The listing builds one solid part. Answer for the finished solid, in the listing's coordinates (mm). Coordinates: 2 decimals unless noted, no trailing zeros. Write each loop counter-clockwise with the first axis right and the second up, starting at its lowest first coordinate (ties: lowest second). Pieces come first, ordered by that corner, then holes.
Autodesk Inventor part; units mm, degrees
ref_plane "YZ Plane" through (0, 0, 0) normal (1, 0, 0) x (0, 1, 0)
ref_plane "XZ Plane" through (0, 0, 0) normal (0, 1, 0) x (-1, 0, 0)
ref_plane "XY Plane" through (0, 0, 0) normal (0, 0, 1) x (1, 0, 0)
sketch "Sketch1" plane through (0, 0, 0) normal (0, 0, 1) x (1, 0, 0)
  circle A0 centre (0, 0) radius 14.5
  dimension "d6" = 29
extrude "Extrusion3" add sketch "Sketch1" along normal blind 300
sketch "Sketch3" plane through (0, 0, 0) normal (1, 0, 0) x (0, 1, 0)
  line L0 (-7, 295.5461) -> (7, 295.5461)
  line L1 (7, 295.5461) -> (7, 320)
  line L2 (7, 320) -> (-7, 320)
  line L3 (-7, 320) -> (-7, 295.5461)
  line L4 (0, 384) -> (0, -64)
  line L5 (14.5, 300) -> (-14.5, 300)
  point P0 (0, 0)
  point P1 (7, 300)
  point P2 (-7, 300)
  dimension "d9" = 7
  dimension "d10" = 7
  dimension "d11" = 20
extrude "Extrusion4" add sketch "Sketch3" along normal mid plane 10 contours L3 L2 L4 L5 | L4 L2 L1 L5
fillet "Fillet1" radius 2 2 edges at (0, -7, 300) (0, 7, 300)
fillet "Fillet2" radius 5 2 edges at (0, -7, 320) (0, 7, 320)
sketch "Sketch4" plane through (5, 0, 0) normal (1, 0, 0) x (0, 0, -1)
  line L0 (-320, 2) -> (-320, -2)
  point P0 (0, 0)
  point P1 (-312, 0)
  dimension "d16" = 8
hole "Hole1" at (5, 0, 312) direction (-1, 0, 0) diameter 8 end through all
equation "\"d10\" = d9"
properties part number "linear_actuator_LH"
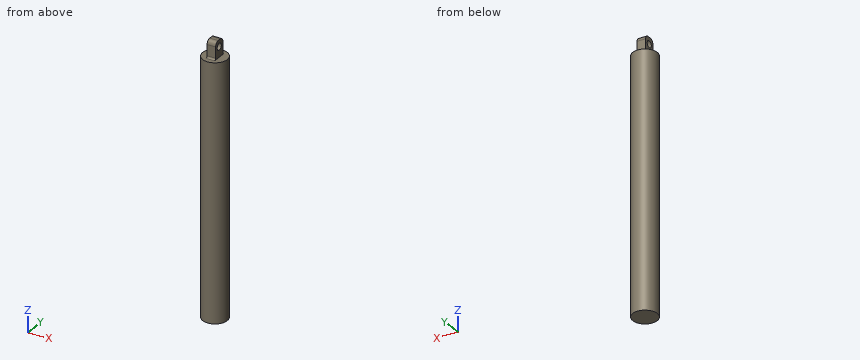
1. Flat-ended cylindrical pins translate along their axes: P1, Ø1, axis at y = 4.5, z = 243.5, coming from the -X side; P2, Ø5, axis at y = 0, z = 312, coming from the +X side; P3, Ø1, axis at y = 2.5, z = 115.5, coming from the +X side; P4, Ø1, axis at x = 2, z = 227.5, coming from the +Y side. Find the tip coordinate at first contact, or state that the pin passes through.
Results found:
P1: stops at x = -13.94
P2: passes through
P3: stops at x = 14.36
P4: stops at y = 14.42
2. Find the intervals of material crossed by L1, parallel to Y at x = -0.5, z = 312; L2, parallel to Z at x = 1, y = 0; L3, parallel to Z at x = -4.25, y = -12.75, in increasing order.
Results found:
L1: y = -7 to -4, 4 to 7
L2: z = 0 to 308, 316 to 320
L3: z = 0 to 300
3. Section A-A on z = 312 is taken. Give the vertices of the cut face in (x, y), then the cut area to 3 significant figures.
Results found:
outline: (-5, -7) - (5, -7) - (5, -4) - (-5, -4) - close; (-5, 4) - (5, 4) - (5, 7) - (-5, 7) - close
area: 60.0 mm2
4. Section B-B on x = 0 is taken. Give the vertices of the cut face in (y, z).
Results found:
outline: (-14.5, 0) - (14.5, 0) - (14.5, 300) - (9, 300) arc R2 cw to (7, 302) - (7, 315) arc R5 ccw to (2, 320) - (-2, 320) arc R5 ccw to (-7, 315) - (-7, 302) arc R2 cw to (-9, 300) - (-14.5, 300) - close; hole circle Ø8 at (0, 312)
5. Section C-C on z = 116 is taken. Give the vertices of the cut face in (x, y), then the cut area to 3 significant figures.
Results found:
outline: circle Ø29 at (0, 0)
area: 661 mm2
